The model under review builds one solid part; all positions refer to its coordinate system, in mm. A direction names the side the tool comes from. Give positions to 0.01 mm unless a question says otherwise; leave off trailing zeros. Write each loop counter-clockwise with the first axis right and the second up, starting at its lowest first coordinate (ties: lowest second). Pieces come first, ordered by that corner, then holes. Notation, with made-up numbers: (71.25, -35.5) -> (109.25, -35.5) arc R29 cw to (109.25, -12.5) -> close; hole circle Ø9 at (-7, -12). An arc over 180 degrees is marked (long way). Use CSV: the item, a comma, the result in double quotes.
```python
from build123d import *

# Parameters (mm, degrees)
PAD_DEPTH    = 2
SKETCH_R     = 3
PAD001_DEPTH = 34


with BuildPart() as part:
    # Sketch001 → Pad (new body, symmetric)
    with BuildSketch(Plane(origin=(0, 0, 0), x_dir=(1, 0, 0), z_dir=(0, 0, -1))):
        Polygon((5.773503, 0), (2.886751, 5), (-2.886751, 5), (-5.773503, 0), (-2.886751, -5), (2.886751, -5), align=None)
    extrude(amount=PAD_DEPTH, both=True)

    # Sketch (on Face7 of Pad) → Pad001 (join)
    with BuildSketch(Plane.XY.offset(2)):
        Circle(SKETCH_R)
    extrude(amount=PAD001_DEPTH)

    # Sketch002 → Groove (revolve, cut)
    with BuildSketch(Plane.XZ):
        Polygon((5.085171, 2.155414), (6.147601, 1.092984), (6.147601, -1.092984), (5.085171, -2.155414), (6.90312, -2.155414), (6.90312, 2.155414), align=None)
    revolve(axis=Axis((0, 0, 0), (0, 0, 1)), mode=Mode.SUBTRACT)


solid = part.part
```
Q1. Machinability: for faces 5 (the conical face through (2.68, -4.68, 1.85)), 6 (the flat face through (2.3, 2.2, 2)), which of the approach directions +Z, -Z, +X, -X, +Y, -Y give a long, thin tool a straight path to every point of the face, cutting with its end or side? Answer none if there is none.
Derived:
face 5,"+Z, +X, -Y"
face 6,"+Z"
Q2. Consider section D-D (x = -4). Write out the cut boundary in (y, z), then the cut area to 3 significant figures.
Derived:
outline,"(-3.07, -2) -> (3.07, -2) -> (3.07, 2) -> (-3.07, 2) -> close"
area,"24.6 mm2"
Q3. The part is to be moulded in two halves that separate along Y. For faces 1 (the cylindrical face through (-3, 0, 19)), 2 (the flat face through (0, 0, 36)), 3 (the conical face through (2.71, 4.66, 1.85)), 4 (the conical face through (-2.707, -4.655, -1.856)), say which applies: pulls with the +Y half, pulls with the -Y half, needs draft (parallel to the pull), parting line crosses it, or undercut.
Derived:
face 1,"parting line crosses it"
face 2,"needs draft"
face 3,"pulls with the +Y half"
face 4,"pulls with the -Y half"
Q4. Insertion check: pin 1 (2 mm diameter, centred on x = -2, z = 20, fed in from -Y); pin 2 (5 mm diameter, centred on y = -3.5, z = 7.5, fed in from -X); pin 3 (1 mm diameter, centred on y = 4, z = 27, fed in from -X); pin 4 (1.5 mm diameter, centred on y = -1.5, z = 19.5, fed in from +X). Each pin has a flat end and moves straight along its axis. Give the tip position at first contact, or say it passes through.
Derived:
pin 1,"stops at y = -2.83"
pin 2,"stops at x = -2.83"
pin 3,"passes through"
pin 4,"stops at x = 2.9"
Q5. Consider section C-C (z = 14). Write out the cut boundary in (x, y), then the cut area to 3 significant figures.
Derived:
outline,"circle Ø6 at (0, 0)"
area,"28.3 mm2"
Q6. Consider section A-A (x = 0). Write out the cut boundary in (y, z), then the cut area to 3 significant figures.
Derived:
outline,"(-5, -2) -> (5, -2) -> (5, 2) -> (3, 2) -> (3, 36) -> (-3, 36) -> (-3, 2) -> (-5, 2) -> close"
area,"244 mm2"
Q7. To check wall thickness, follow probe 1 along Z at (x, y) = (-1.5, 3.25); probe 2 along X at (y, z) = (-0.5, 12); probe 3 along Y at (x, z) = (-1.5, 31.5). State the ranges of each line that lie inside material, in increasing order.
Derived:
probe 1,"z = -2 to 2"
probe 2,"x = -2.96 to 2.96"
probe 3,"y = -2.6 to 2.6"
Q8. Consider section B-B (y = 2). Write out the cut boundary in (x, z), then the cut area to 3 significant figures.
Derived:
outline,"(-4.62, -2) -> (4.62, -2) -> (4.62, 2) -> (2.24, 2) -> (2.24, 36) -> (-2.24, 36) -> (-2.24, 2) -> (-4.62, 2) -> close"
area,"189 mm2"
